Autodesk Inventor part; units mm, degrees
ref_plane "YZ Plane" through (0, 0, 0) normal (1, 0, 0) x (0, 1, 0)
ref_plane "XZ Plane" through (0, 0, 0) normal (0, 1, 0) x (-1, 0, 0)
ref_plane "XY Plane" through (0, 0, 0) normal (0, 0, 1) x (1, 0, 0)
sketch "Sketch1" plane through (0, 0, 0) normal (1, 0, 0) x (0, 1, 0)
  line L0 (90, 0) -> (0, 0) construction
  line L1 (0, 0) -> (0, -135) construction
  line L2 (0, -135) -> (90, -135) construction
  line L3 (90, -135) -> (90, 0) construction
  line L4 (80, 0) -> (65, 0)
  line L5 (80, 0) -> (90, -18.1711)
  line L6 (90, -18.1711) -> (87.7664, -82.1322)
  line L7 (87.7664, -82.1322) -> (61.6218, -109.7086)
  line L8 (2.8311, -135) -> (0, -119.8888)
  line L9 (52.695, -83.5675) -> (60.7393, -49.8037)
  line L10 (60.7393, -49.8037) -> (55.0089, -17.3051)
  line L11 (55.0089, -17.3051) -> (65, 0)
  line L12 (55.0089, -17.3051) -> (52.695, -83.5675) construction
  line L13 (52.695, -83.5675) -> (0, -119.8888)
  line L14 (2.8311, -135) -> (61.6218, -109.7086)
  line L15 (87.7664, -82.1322) -> (0, -119.8888) construction
  line L16 (80, 0) -> (61.6218, -109.7086) construction
  line L17 (0, 27) -> (0, -162)
  line L18 (-18, 0) -> (108, 0)
  circle A0 centre (77.4826, -15.0279) radius 2
  circle A1 centre (63.4392, -98.8597) radius 2
  line L19 (61.6218, -109.7086) -> (23.93, -103.3945) construction
  dimension "d10" = 135
  dimension "d11" = 90
  dimension "d29" = 10
  dimension "d30" = 15
  dimension "d31" = 2
  dimension "d34" = 120
  dimension "d37" = 64
  dimension "d39" = 35
  dimension "d40" = 140
  dimension "d42" = 38
  dimension "d43" = 15
  dimension "d44" = 64
  dimension "d45" = 64
  dimension "d46" = 33
  dimension "d47" = 34.7088
  dimension "d59" = 85
  dimension "d60" = 11
  dimension "d61" = 4
extrude "Extrusion1" add sketch "Sketch1" along normal blind 14 contours L5 L6 L7 L14 L8 L13 L9 L10 L11 L4
sketch "Sketch2" plane through (0, 0, 0) normal (-1, 0, 0) x (0, 0, 1)
  line L0 (-18.1711, 90) -> (0, 80)
  line L1 (-82.1322, 87.7664) -> (-18.1711, 90)
  line L2 (-109.7086, 61.6218) -> (-82.1322, 87.7664)
  line L3 (-135, 2.8311) -> (-109.7086, 61.6218)
  line L4 (-119.8888, 0) -> (-135, 2.8311)
  line L5 (-83.5675, 52.695) -> (-119.8888, 0)
  line L6 (-49.8037, 60.7393) -> (-83.5675, 52.695)
  line L7 (-17.3051, 55.0089) -> (-49.8037, 60.7393)
  line L8 (0, 65) -> (-17.3051, 55.0089)
  line L9 (0, 80) -> (0, 65)
  circle A0 centre (-98.8597, 63.4392) radius 2
  circle A1 centre (-15.0279, 77.4826) radius 2
  line L10 (-135, 2.8311) -> (-109.7086, 61.6218)
  line L11 (-18.1711, 90) -> (0, 80)
  line L12 (-5.748, 62.8835) -> (-60.8643, 86.5942)
  line L13 (-60.8643, 86.5942) -> (-108.2857, -23.6383)
  line L14 (-108.2857, -23.6383) -> (-53.1695, -47.349)
  line L15 (-53.1695, -47.349) -> (-5.748, 62.8835)
  line L16 (-18.1711, 90) -> (-27.3572, 93.9518)
  point P0 (-74.5203, 54.8505)
  point P1 (-6.436, 61.2841)
  dimension "d70" = 35
  dimension "d72" = 120
  dimension "d76" = 60
  dimension "d78" = 10
  dimension "d79" = 20
extrude "Extrusion2" add sketch "Sketch2" along normal blind 40 and the other way blind 50 contours L15 L14 L13 L6 L7 L8 | L8 L7 L6 L13 L12 L15
sketch "Sketch3" plane through (-40, 0, 0) normal (-1, 0, 0) x (0, 0, 1)
  circle A0 centre (-15.0279, 77.4826) radius 2
  line L0 (-83.5675, 52.695) -> (-15.0279, 77.4826)
  line L1 (-5.748, 62.8835) -> (-60.8643, 86.5942)
  line L2 (-60.8643, 86.5942) -> (-108.2857, -23.6383)
  line L3 (-5.748, 62.8835) -> (-53.1695, -47.349)
  line L4 (-29.4587, 7.7672) -> (-84.575, 31.4779) construction
  line L5 (-99.2863, 16.1562) -> (-70.1502, -50.6509)
  line L6 (-108.2857, -23.6383) -> (-53.1695, -47.349)
  point P0 (0, 0)
  point P1 (-73.9515, 56.1726)
  point P2 (-28.423, 72.6381)
  point P3 (-75.8445, -37.5944)
  point P4 (-95.1985, 6.7833)
extrude "Extrusion3" cut sketch "Sketch3" against normal up to surface (40 mm away) contours L0 L2 L1 | L5 L6 L2
sketch "Sketch4" plane through (50, 0, 0) normal (1, 0, 0) x (0, 0, -1)
  line L0 (5.748, 62.8835) -> (60.8643, 86.5942)
  line L1 (60.8643, 86.5942) -> (108.2857, -23.6383)
  line L2 (28.423, 72.6381) -> (73.9515, 56.1726)
  line L3 (99.2863, 16.1562) -> (70.1502, -50.6509)
  line L4 (108.2857, -23.6383) -> (53.1695, -47.349)
  point P0 (0, 0)
  point P1 (75.8445, -37.5944)
  point P2 (95.1985, 6.7833)
extrude "Extrusion4" cut sketch "Sketch4" against normal up to surface (36 mm away)
sketch "Sketch5" plane through (14, 0, 0) normal (-1, 0, 0) x (0, 0, 1)
  circle A0 centre (-158.0633, 63.0922) radius 125
  line L0 (-29.4587, 7.7672) -> (-84.575, 31.4779) construction
  line L1 (-84.575, 31.4779) -> (-158.0633, 63.0922)
  point P0 (0, 0)
  dimension "d88" = 80
  dimension "d89" = 250
extrude "Extrusion5" cut sketch "Sketch5" against normal blind 7
equation "\"d61\" = Mount_Hole_Diameter"
equation "\"Mount_Hole_Diameter\" = 4"
properties part number "F3 Front Caliper Bracket"
The listing builds one solid part. Answer for the finished solid, in the listing's coordinates (mm). A direction names the side the tool comes from. Round coordinates to 2 decimals unless told otherwise and drop trailing zeros. Loops run counter-clockwise (first coordinate to the right, second up) from the corner with the lowest first, then second, coordinate; pieces in that order, holes last. Notation, with made-up numbers: M 68.5,20 L 85.5,20 A21 cw 85.5,56 Z; hole C 75,-38.5 d10. An arc over 180 degrees is marked long. Return JSON: item names as keys, results as strings.
Q1. Find section A-A, the plane y = 16.5. Determine the outline of the cut face in (x, z), plus the area to 3 significant figures.
Results list:
{"outline": "M -40,-91.02 L 14,-91.02 L 14,-42.07 L 21,-42.07 L 21,-91.02 L 50,-91.02 L 50,-25.7 L -40,-25.7 Z; M 0,-129.12 L 14,-129.12 L 14,-108.52 L 0,-108.52 Z", "area": "5,820 mm2"}
Q2. Which of the six approach directions +Z, -Z, +X, -X, +Y, -Y give full straight-line access (tool end or side, diameter ignored) to faces 1 (the face through (-20.28, -15.09, -85.66)), 2 (the face through (36.25, 64.52, -50.87)), 3 (the face through (36.25, -15.09, -85.66)), 4 (the face through (-20.28, 64.29, -51.51)), 5 (the face through (-19.72, 67.693, -16.927))?
Results list:
{"face 1": "-Z, -X, -Y", "face 2": "-Z, +X, +Y", "face 3": "-Z, +X, -Y", "face 4": "-Z, -X, +Y", "face 5": "+Z, -X, +Y"}
Q3. The mould has two halves that part along Y. Classify faces 6 (the face through (-12.622, 25.694, -87.063)), 7 (the face through (5.63, 7, -29.79)), 8 (the face through (14, 39, -67)): released by +Y, released by -Y, zero draft, split by the parting line, or undercut.
Results list:
{"face 6": "undercut", "face 7": "released by -Y", "face 8": "zero draft"}
Q4. Find the intervals of material crossed by line 1 along X through (y, z) = (-8.5, -79.5); line 2 along X through (y, z) = (81, -7.5); line 3 along Z through (x, y) = (8, 30), in increasing order. Write a range as from..to.
Results list:
{"line 1": "x = -40..14, 21..50", "line 2": "x = 0..14", "line 3": "z = -123.31..-99.21, -85.21..-19.89"}
Q5. Find section C-C, the plane x = 10. Determine the outline of the cut face in (y, z) (1 decimal), plus the area to 3 significant figures.
Results list:
{"outline": "M -47.3,-53.2 L -23.6,-108.3 L 54.9,-74.5 L 52.7,-83.6 L 0,-119.9 L 2.8,-135 L 61.6,-109.7 L 87.8,-82.1 L 90,-18.2 L 80,0 L 65,0 L 61.3,-6.4 Z; hole C 63.4,-98.9 d4; hole C 77.5,-15 d4", "area": "10,400 mm2"}
Q6. Each of these flat-tipped pins is pushed along its axis until it touches: pin 1 Ø2 at (x, y) = (29.5, -23) entering from -Z; pin 2 Ø2 at (y, z) = (47, -118) entering from -X; pin 3 Ø12 at (x, z) = (17.5, -99.5) entering from +Y; pin 4 Ø6.5 at (y, z) = (63.44, -98.86) entering from +X. Where does it stop, or does it pass through?
Results list:
{"pin 1": "stops at z = -82.65", "pin 2": "passes through", "pin 3": "stops at y = 75.92", "pin 4": "stops at x = 14"}
Q7. Find section D-D, the plane y = -7. Determine the outline of the cut face in (x, z).
Results list:
{"outline": "M -40,-89.19 L 0,-89.19 L 0,-101.13 L 14,-101.13 L 14,-54.56 L 21,-54.56 L 21,-89.19 L 50,-89.19 L 50,-35.81 L -40,-35.81 Z"}
Q8. Find section B-B, the plane z = -93. Determine the outline of the cut face in (x, y), plus the area to 3 significant figures.
Results list:
{"outline": "M -40,1.74 L 0,1.74 L 0,-30.21 L 14,-30.21 L 14,11.89 L -40,11.89 Z; M 0,39.01 L 14,39.01 L 14,77.46 L 0,77.46 Z; M 21,1.74 L 50,1.74 L 50,11.89 L 21,11.89 Z", "area": "1,830 mm2"}
